Autodesk Inventor part; units mm, degrees
ref_plane "YZ Plane" through (0, 0, 0) normal (1, 0, 0) x (0, 1, 0)
ref_plane "XZ Plane" through (0, 0, 0) normal (0, 1, 0) x (-1, 0, 0)
ref_plane "XY Plane" through (0, 0, 0) normal (0, 0, 1) x (1, 0, 0)
sketch "Sketch9" plane through (0, 0, 0) normal (0, 1, 0) x (-1, 0, 0)
  line L0 (15, 15) -> (-15, 15)
  line L1 (-15, 15) -> (-15, -15)
  line L2 (-15, -15) -> (15, -15)
  line L3 (15, -15) -> (15, 15)
  line L4 (15, 15) -> (-15, -15) construction
  line L5 (-15, 15) -> (15, -15) construction
  line L6 (-13, 13) -> (13, 13)
  line L7 (13, 13) -> (13, -13)
  line L8 (13, -13) -> (-13, -13)
  line L9 (-13, -13) -> (-13, 13)
  point P0 (0, 0)
  dimension "d172" = 30
  dimension "d173" = 30
  dimension "d174" = 2
extrude "Extrusion3" add sketch "Sketch9" against normal blind 225
sketch "Sketch10" plane through (0, 0, 0) normal (1, 0, 0) x (0, 1, 0)
  line L0 (0, 15) -> (0, -15) construction
  line L1 (0, 15) -> (-225, 15) construction
  line L2 (0, -15) -> (-225, -15) construction
  line L3 (-58.5, 8.5) -> (-41.5, 8.5)
  line L4 (-41.5, 8.5) -> (-41.5, -8.5)
  line L5 (-41.5, -8.5) -> (-58.5, -8.5)
  line L6 (-58.5, -8.5) -> (-58.5, 8.5)
  line L7 (-58.5, 8.5) -> (-41.5, -8.5) construction
  line L8 (-41.5, 8.5) -> (-58.5, -8.5) construction
  line L9 (0, 0) -> (30, 0)
  circle A0 centre (-50, 0) radius 8.5
  dimension "d177" = 17
  dimension "d178" = 17
  dimension "d181" = 30
  dimension "d182" = 80
extrude "Extrusion4" cut sketch "Sketch10" along normal through all contours A0
pattern_linear "Rectangular Pattern4" count 4 spacing 68 along (0, -1, 0) of "Extrusion4"
properties part number "PRS 1662 DrSysB way tube 44_D1200" material "Stainless Steel"
Build history of the part. All positions in model axes, mm. A direction names the side the tool comes from. Coordinates: 2 decimals unless noted, no trailing zeros. Order: outer loops, then holes, each group sorted by start corner. A loop starts at its lowest first (then second) coordinate and runs counter-clockwise, first axis right, second up.
Item 1: Saw through at A-A on z = 0. List the corners of the cut face in (x, y).
Filled in:
outline: (-15, -225) - (-13, -225) - (-13, 0) - (-15, 0) - close; (13, -225) - (15, -225) - (15, -194.5) - (13, -194.5) - close; (13, -177.5) - (15, -177.5) - (15, -126.5) - (13, -126.5) - close; (13, -109.5) - (15, -109.5) - (15, -58.5) - (13, -58.5) - close; (13, -41.5) - (15, -41.5) - (15, 0) - (13, 0) - close
Item 2: Mould opens along Y. For faces 1 (the flat face through (0, -111, -13)), 2 (the flat face through (14, 0, 0)), 3 (the cylindrical face through (13.986, -56.265, -5.745)) say: released by +Y, released by -Y, zero draft, split by the parting line, or undercut.
Filled in:
face 1: zero draft
face 2: released by +Y
face 3: undercut
Item 3: Saw through at B-B on y = -206. List the corners of the cut face in (x, z).
Filled in:
outline: (-15, -15) - (15, -15) - (15, 15) - (-15, 15) - close; hole (-13, -13) - (13, -13) - (13, 13) - (-13, 13) - close
Item 4: Drop a flat-ended pin along its axis: pin 1 Ø13.5 at (y, z) = (-50, 0) entering from +X. Give the stop position or say it passes through.
Filled in:
pin 1: stops at x = -13
Item 5: Saw through at D-D on z = -11. List the corners of the cut face in (x, y).
Filled in:
outline: (-15, -225) - (-13, -225) - (-13, 0) - (-15, 0) - close; (13, -225) - (15, -225) - (15, 0) - (13, 0) - close
Item 6: Saw through at C-C on x = 7. List the corners of the cut face in (y, z), then the cut area to 3 significant figures.
Filled in:
outline: (-225, -15) - (0, -15) - (0, -13) - (-225, -13) - close; (-225, 13) - (0, 13) - (0, 15) - (-225, 15) - close
area: 900 mm2
Item 7: Drill centre lines: L1, parallel to Y at x = 14.5, z = 0; L2, parallel to X at y = -169.5, z = 11.5. Where is each one in solid material? Low to high.
Filled in:
L1: y = -225 to -194.5, -177.5 to -126.5, -109.5 to -58.5, -41.5 to 0
L2: x = -15 to -13, 13 to 15
Item 8: Tool access for faces 4 (the flat face through (13, -111, -6)), 5 (the flat face through (0, -111, 15)), 6 (the cylindrical face through (13.99, -109.89, -2.55)): list every direction of +Z, -Z, +X, -X, +Y, -Y with a clear straight run to the whole face (end or side of a thin tool).
Filled in:
face 4: +Y, -Y
face 5: +Z, +X, -X, +Y, -Y
face 6: +X
